```python
from build123d import *

# Parameters (mm, degrees)
SKETCH_1_W      = 72.5
SKETCH_1_H      = 87.5
SKETCH_1_R      = 1.6
SKETCH_1_W_2    = 42.5
SKETCH_1_H_2    = 57.5
EXTRUDE_1_DEPTH = 2
FILLET_1_R      = 5


with BuildPart() as part:
    # 草图1 → 凸台-拉伸1 (new body)
    with BuildSketch(Plane(origin=(0, 0, 0), x_dir=(1, 0, 0), z_dir=(0, 1, 0))):
        with Locations((21.25, 28.75)):
            Rectangle(SKETCH_1_W, SKETCH_1_H)
        with Locations(Location((-7.6, 65, 0), (0, 0, 270))):
            Circle(SKETCH_1_R, mode=Mode.SUBTRACT)
        with Locations(Location((21.25, 65, 0), (0, 0, 270))):
            Circle(SKETCH_1_R, mode=Mode.SUBTRACT)
        with Locations(Location((50.1, 65, 0), (0, 0, 270))):
            Circle(SKETCH_1_R, mode=Mode.SUBTRACT)
        with Locations(Location((50.1, -7.5, 0), (0, 0, 270))):
            Circle(SKETCH_1_R, mode=Mode.SUBTRACT)
        with Locations(Location((21.25, -7.5, 0), (0, 0, 270))):
            Circle(SKETCH_1_R, mode=Mode.SUBTRACT)
        with Locations(Location((-7.6, -7.5, 0), (0, 0, 270))):
            Circle(SKETCH_1_R, mode=Mode.SUBTRACT)
        with Locations(Location((-5, 45, 0), (0, 0, 270))):
            Circle(SKETCH_1_R, mode=Mode.SUBTRACT)
        with Locations(Location((-5, 12.5, 0), (0, 0, 270))):
            Circle(SKETCH_1_R, mode=Mode.SUBTRACT)
        with Locations(Location((47.5, 12.5, 0), (0, 0, 90))):
            Circle(SKETCH_1_R, mode=Mode.SUBTRACT)
        with Locations(Location((47.5, 45, 0), (0, 0, 90))):
            Circle(SKETCH_1_R, mode=Mode.SUBTRACT)
        with Locations((21.25, 28.75)):
            Rectangle(SKETCH_1_W_2, SKETCH_1_H_2, mode=Mode.SUBTRACT)
    extrude(amount=EXTRUDE_1_DEPTH)

    # 圆角1
    fillet_1_edges = [part.edges().sort_by_distance(p)[0] for p in [
        (0, 1, -57.5),
        (0, 1, 0),
        (42.5, 1, 0),
        (42.5, 1, -57.5),
        (-15, 1, 15),
        (-15, 1, -72.5),
        (57.5, 1, -72.5),
        (57.5, 1, 15),
    ]]
    fillet(fillet_1_edges, radius=FILLET_1_R)


solid = part.part
```
Source: CAD feature listing. Evaluate the final solid. Frame: model axes, mm. A direction names the side the tool comes from. Coordinates: 2 decimals unless noted, no trailing zeros. Order: outer loops, then holes, each group sorted by start corner. A loop starts at its lowest first (then second) coordinate and runs counter-clockwise, first axis right, second up. Notation, with made-up numbers: M 47,-17.75 L 62,-17.75 A10 cw 62,-5.75 Z; hole C -0.75,6.25 d10. An arc over 180 degrees is marked long. Write each question's results on one line, items separated by ' | '. Start each with the question number.
1) Section query C-C (x = 47.5). Return the cut outline in (y, z), plus the area to 3 significant figures.
2) Draft query along X for faces 1 (the face through (41, 1.01, -1.43)), 2 (the face through (-14, 1, 13)), 3 (the face through (21, 1, -72.5)). Return one class per face: released by +X, released by -X, zero draft, split by the parting line, or undercut.
3) Section query B-B (x = 25.5). Return the cut outline in (y, z), plus the area to 3 significant figures.
4) Section query A-A (z = -45). Return the cut outline in (x, y).
5) Line query: line 1 (Z direction, x = -7.5, y = 1.2); line 2 (X direction, y = 1.45, z = 7.5); line 3 (Z direction, x = 36, y = 1.9). Output: solid intervals per line, ascending. Write a range as from..to.
6) Section query D-D (y = 1.65). Give the number of separate pieces and of enclosed holes in the cut face, plus the area to 3 significant figures.
7) Contact query for a flat-ended pin moving along its axis: pin 1 Ø4 at (x, z) = (21.25, 7.5) entering from +Y. Output: stop coordinate, or through.
8) Access query for faces 4 (the face through (-13.57, 1.01, -71)), 5 (the face through (21, 1, 0)). Directions: +Z, -Z, +X, -X, +Y, -Y. A direction counts if a zero-diameter tool reaches every point of the face in a straight line with its end or side. Return the directions, or none.
Answers:
1) outline: M 0,-72.5 L 2,-72.5 L 2,-46.6 L 0,-46.6 Z; M 0,-43.4 L 2,-43.4 L 2,-14.1 L 0,-14.1 Z; M 0,-10.9 L 2,-10.9 L 2,15 L 0,15 Z | area: 162 mm^2
2) face 1: undercut | face 2: released by -X | face 3: zero draft
3) outline: M 0,-72.5 L 2,-72.5 L 2,-57.5 L 0,-57.5 Z; M 0,0 L 2,0 L 2,15 L 0,15 Z | area: 60.0 mm^2
4) outline: M -15,0 L -6.6,0 L -6.6,2 L -15,2 Z; M -3.4,0 L 0,0 L 0,2 L -3.4,2 Z; M 42.5,0 L 45.9,0 L 45.9,2 L 42.5,2 Z; M 49.1,0 L 57.5,0 L 57.5,2 L 49.1,2 Z
5) line 1: z = -72.5..-66.6, -63.4..5.9, 9.1..15 | line 2: x = -15..-9.2, -6..19.65, 22.85..48.5, 51.7..57.5 | line 3: z = -72.5..-57.5, 0..15
6) separate pieces: 1 | enclosed holes: 11 | area: 3,820 mm^2
7) pin 1: stops at y = 2
8) face 4: -Z, -X, +Y, -Y | face 5: +Y, -Y
